Input: part model. Units: mm. Frame: model coordinates. Face numbers are marked on the shaded views. A direction names the side the tool comes from. Round coordinates to 2 decimals unless told otherwise and drop trailing zeros. Order: outer loops, then holes, each group sorted by start corner. A loop starts at its lowest first (then second) coordinate and runs counter-clockwise, first axis right, second up. Notation, with made-up numbers: (50, -10) -> (75, -10) arc R21 cw to (75, -1) -> close; hole circle Ø9 at (79.25, -37.75). An arc over 180 degrees is marked (long way). Use a Markdown table: item, result.
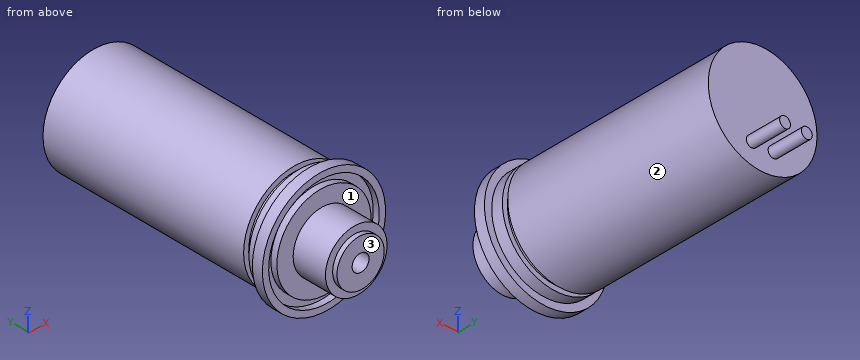
from build123d import *

# Parameters (mm, degrees)
SKETCH2_R           = 0.75
BOSS_EXTRUDE1_DEPTH = 5
SKETCH3_W           = 0.99
SKETCH3_H           = 0.65
SKETCH4_R           = 1.17
CUT_EXTRUDE1_DEPTH  = 7.5
SKETCH5_W           = 1.13
SKETCH5_H           = 0.9
SKETCH_N_W          = 0.8
SKETCH_N_H          = 0.8


with BuildPart() as part:
    # Sketch1 → Revolve2 (revolve)
    with BuildSketch(Plane.XY):
        Polygon((0, 0), (-4.25, 0), (-4.25, 5.5), (-8.5, 5.5), (-8.5, 7), (-7.5, 7), (-7.5, 39.5), (0, 39.5), align=None)
    revolve(axis=Axis((0, 0, 0), (0, 1, 0)))

    # Sketch2 → Boss-Extrude1 (add)
    with BuildSketch(Plane(origin=(0, 39.5, 0), x_dir=(1, 0, 0), z_dir=(0, 1, 0))):
        with Locations((1.5, 4.5)):
            Circle(SKETCH2_R)
        with Locations((-1.5, 4.5)):
            Circle(SKETCH2_R)
    extrude(amount=BOSS_EXTRUDE1_DEPTH)

    # Sketch3 → Cut-Revolve1 (revolve, cut)
    with BuildSketch(Plane(origin=(0, 0, 0), x_dir=(0, 0, -1), z_dir=(1, 0, 0))):
        with Locations((3.755, 0.325)):
            Rectangle(SKETCH3_W, SKETCH3_H)
    revolve(axis=Axis((0, 0, 0), (0, 1, 0)), mode=Mode.SUBTRACT)

    # Sketch4 → Cut-Extrude1 (cut)
    with BuildSketch(Plane.XZ):
        Circle(SKETCH4_R)
    extrude(amount=-CUT_EXTRUDE1_DEPTH, mode=Mode.SUBTRACT)

    # Sketch5 → Cut-Revolve2 (revolve, cut)
    with BuildSketch(Plane(origin=(0, 0, 0), x_dir=(0, 0, -1), z_dir=(1, 0, 0))):
        with Locations((7.065, 5.95)):
            Rectangle(SKETCH5_W, SKETCH5_H)
    revolve(axis=Axis((0, 0, 0), (0, 1, 0)), mode=Mode.SUBTRACT)

    # Sketch N → Cut-Revolve8 (revolve, cut)
    with BuildSketch(Plane(origin=(0, 0, 0), x_dir=(0, 0, -1), z_dir=(1, 0, 0))):
        with Locations((7.2, 9)):
            Rectangle(SKETCH_N_W, SKETCH_N_H)
    revolve(axis=Axis((0, 0, 0), (0, 1, 0)), mode=Mode.SUBTRACT)


solid = part.part
1) Cut plane D-D on y = 19. Return loops of the section in (x, z), and give its area (3 significant figures).
Answer key:
| item | result |
|---|---|
| outline | circle Ø15 at (0, 0) |
| area | 177 mm^2 |
2) Set-up query: the marked faces 1, 2 and 3. Return all of +Z, -Z, +X, -X, +Y, -Y with unobstructed straight access to the full face (end or side cutting, diameter ignored); none if empty.
Answer key:
| item | result |
|---|---|
| face 1 | -Y |
| face 2 | +Y |
| face 3 | +Z, -Z, +X, -X, -Y |
3) Ray query, probe 1 along Z at (x, y) = (0, 6.25); probe 2 along Y at (x, z) = (-1.75, 7.25); probe 3 along Y at (x, z) = (3.5, 0.5). Return the intervals inside material, ascending.
Answer key:
| item | result |
|---|---|
| probe 1 | z = -8.5 to -7.63, -6.5 to -1.17, 1.17 to 6.5, 7.63 to 8.5 |
| probe 2 | y = 6.4 to 8.6, 9.4 to 39.5 |
| probe 3 | y = 0.65 to 39.5 |
4) Cut plane B-B on x = 5.25. Return loops of the section in (y, z), and give its area (3 significant figures).
Answer key:
| item | result |
|---|---|
| outline | (5.5, -6.68) -> (7, -6.68) -> (7, -5.36) -> (8.6, -5.36) -> (8.6, -4.32) -> (9.4, -4.32) -> (9.4, -5.36) -> (39.5, -5.36) -> (39.5, 5.36) -> (9.4, 5.36) -> (9.4, 4.32) -> (8.6, 4.32) -> (8.6, 5.36) -> (7, 5.36) -> (7, 6.68) -> (5.5, 6.68) -> (5.5, 5.54) -> (6.4, 5.54) -> (6.4, 3.83) -> (5.5, 3.83) -> (5.5, -3.83) -> (6.4, -3.83) -> (6.4, -5.54) -> (5.5, -5.54) -> close |
| area | 363 mm^2 |
5) Cut plane C-C on z = 3.75. Return loops of the section in (x, y).
Answer key:
| item | result |
|---|---|
| outline | (-7.63, 5.5) -> (-6.64, 5.5) -> (-6.64, 6.4) -> (-5.31, 6.4) -> (-5.31, 5.5) -> (-2, 5.5) -> (-2, 0.65) -> (2, 0.65) -> (2, 5.5) -> (5.31, 5.5) -> (5.31, 6.4) -> (6.64, 6.4) -> (6.64, 5.5) -> (7.63, 5.5) -> (7.63, 7) -> (6.5, 7) -> (6.5, 8.6) -> (5.67, 8.6) -> (5.67, 9.4) -> (6.5, 9.4) -> (6.5, 39.5) -> (-6.5, 39.5) -> (-6.5, 9.4) -> (-5.67, 9.4) -> (-5.67, 8.6) -> (-6.5, 8.6) -> (-6.5, 7) -> (-7.63, 7) -> close |
6) Cut plane A-A on y = 40.5. Return loops of the section in (x, z).
Answer key:
| item | result |
|---|---|
| outline | circle Ø1.5 at (-1.5, -4.5); circle Ø1.5 at (1.5, -4.5) |
7) Contact query for flat-ended pins moving along their axis: P1, Ø5, axis at x = -6, y = 27, coming from the +Z side; P2, Ø3, axis at x = 5.5, z = -1.5, coming from the +Y side; P3, Ø8, axis at x = -3.5, y = 33, coming from the -Z side. Output: stop coordinate, or through.
Answer key:
| item | result |
|---|---|
| P1 | stops at z = 6.63 |
| P2 | stops at y = 39.5 |
| P3 | stops at z = -7.5 |
